Here's how the part is built. I have some questions about the finished solid (model axes, mm). A direction names the side the tool comes from. Round coordinates to 2 decimals unless told otherwise and drop trailing zeros. Loops run counter-clockwise (first coordinate to the right, second up) from the corner with the lowest first, then second, coordinate; pieces in that order, holes last. Notation, with made-up numbers: M -34.75,21 L -9.75,21 A15 ccw -9.75,49 Z; hole C 11,-30 d1. An arc over 180 degrees is marked long. Answer as a JSON object with one key per item and string values.
from build123d import *

# Parameters (mm, degrees)
F1_DEPTH = 11.1125
F2_R     = 0.254
F3_R     = 6.737778
F4_DEPTH = 9.525
F5_W     = 6.35
F5_H     = 6.35
F6_DEPTH = 6.604


with BuildPart() as f1:
    # F0 (on Top) → F1 (new body)
    with BuildSketch(Plane.XY):
        with BuildLine():
            ThreePointArc((4.7625, 4.5085), (4.688105, 4.688105), (4.5085, 4.7625))
            Line((4.5085, 4.7625), (-4.5085, 4.7625))
            ThreePointArc((-4.5085, 4.7625), (-4.688105, 4.688105), (-4.7625, 4.5085))
            Line((-4.7625, 4.5085), (-4.7625, -4.5085))
            ThreePointArc((-4.7625, -4.5085), (-4.688105, -4.688105), (-4.5085, -4.7625))
            Line((-4.5085, -4.7625), (4.5085, -4.7625))
            ThreePointArc((4.5085, -4.7625), (4.688105, -4.688105), (4.7625, -4.5085))
            Line((4.7625, -4.5085), (4.7625, 4.5085))
        make_face()
    extrude(amount=F1_DEPTH)

    # F2
    f2_edges = [f1.edges().sort_by_distance(p)[0] for p in [
        (4.7625, 0, 0),
    ]]
    fillet(f2_edges, radius=F2_R)

    # F3 (on face) → F4 (join)
    with BuildSketch(Plane.XY.offset(11.1125)):
        Circle(F3_R)
    extrude(amount=F4_DEPTH)

    # F5 (on face) → F6 (cut)
    with BuildSketch(Plane.XY.offset(20.6375)):
        Rectangle(F5_W, F5_H)
    extrude(amount=-F6_DEPTH, mode=Mode.SUBTRACT)


solid = f1.part
Item 1: If we mould it in two halves opening along X, with no side actions, what happens to faces 1 (the face through (-4.762, 0, 6)), 2 (the face through (-3.175, 0, 17)), 3 (the face through (0, -4, 20.638))? For each: pulls with the +X half, pulls with the -X half, needs draft (parallel to the pull), parting line crosses it, or undercut.
Resolved:
{"face 1": "pulls with the -X half", "face 2": "undercut", "face 3": "needs draft"}
Item 2: I'm going to push flat-ended pins straight in: pin 1 Ø1.9 at (y, z) = (-1.5, 18) entering from +X; pin 2 Ø6 at (x, z) = (4, 18) entering from +Y; pin 3 Ø1.9 at (x, y) = (1, 0) entering from +Z; pin 4 Ø8 at (x, y) = (4.5, -1.5) entering from -Z. Where does each tip first touch, or does it pass through?
Resolved:
{"pin 1": "x = 6.72", "pin 2": "y = 6.66", "pin 3": "z = 14.03", "pin 4": "z = 0"}
Item 3: On a 3-axis mill with a long thin cutter (end or side, diameter ignored), from which of +Z, -Z, +X, -X, +Y, -Y can I reach the whole of each face in a straight line? I mean faces 4 (the face through (3.175, 0, 17)), 5 (the face through (0, 4.762, 6)), 6 (the face through (0, -4.762, 6)), 7 (the face through (4.762, 0, 6)). Say none if no direction works.
Resolved:
{"face 4": "+Z", "face 5": "-Z, +X, -X, +Y", "face 6": "-Z, +X, -X, -Y", "face 7": "-Z, +X, +Y, -Y"}
Item 4: Please list where these lines run through material, in increasing order: probe 1 along Y at (x, z) = (0, 17.25) (3 decimals); probe 2 along X at (y, z) = (4, 7.75). Write a range as from..to.
Resolved:
{"probe 1": "-6.738..-3.175, 3.175..6.738", "probe 2": "-4.76..4.76"}
Item 5: I want a section at D-D, the plane z = 3.75. Please give me the cut outline in (x, y).
Resolved:
{"outline": "M -4.76,-4.51 A0.25 ccw -4.51,-4.76 L 4.51,-4.76 A0.25 ccw 4.76,-4.51 L 4.76,4.51 A0.25 ccw 4.51,4.76 L -4.51,4.76 A0.25 ccw -4.76,4.51 Z"}
Item 6: I want a section at C-C, the plane z = 18.25. Please give me the cut outline in (x, y) (3 decimals), then the cut area to 3 significant figures.
Resolved:
{"outline": "C 0,0 d13.476; hole M -3.175,-3.175 L 3.175,-3.175 L 3.175,3.175 L -3.175,3.175 Z", "area": "102 mm²"}
